Input: part model. Units: mm. Frame: model coordinates. Give positions to 0.01 mm unless a question says otherwise; leave off trailing zeros. Loops run counter-clockwise (first coordinate to the right, second up) from the corner with the lowest first, then second, coordinate; pieces in that order, holes last. Notation, with made-up numbers: M 16,18 L 47,18 A23 cw 47,57 Z; hole C 51,-10 d7. An arc over 180 degrees is marked long. One line per item, written item: value. Start each with the question number.
(1) Pin query (flat end, axial travel): P1, Ø11, axis at y = 314.18, z = 1303.08, coming from the -X side; P2, Ø4, axis at y = 259.2, z = 1328.48, coming from the -X side. Return the tip coordinate at first contact, or that it passes through.
(2) Section D-D on z = 1313.5. Output: boundary loops of the cut face in (x, y).
(3) Section C-C on y = 267.5. Output: boundary loops of the cut face in (x, z), plus the area to 3 significant figures.
(4) Section A-A on z = 1277. Output: boundary loops of the cut face in (x, y), plus the area to 3 significant figures.
(5) Section B-B on x = 95.3. Output: boundary loops of the cut face in (y, z) (3 decimals), plus the area to 3 significant figures.
(6) Ray query, line 1 along Z through (x, y) = (95.3, 316.5); line 2 along Y through (x, z) = (95.05, 1278.5); line 3 along Y through (x, z) = (94.45, 1280.5). Return the intervals inside material, ascending. Write a range as from..to.
(7) Pull-direction query (Z, two-part tool) for faces 1 (the cylindrical face through (94.479, 316.098, 1335.797)), 2 (the cylindrical face through (94.43, 284.75, 1325.1)), 3 (the flat face through (96.044, 298, 1310)); classes: released by +Z, released by -Z, zero draft, split by the parting line, or undercut.
```python
from build123d import *

# Parameters (mm, degrees)
BOSS_EXTRUDE1_START     = 92.868812
BOSS_EXTRUDE1_DEPTH     = 3.175
FILLET1_R               = 9.525
F_1_4_CLEARANCE_HOLE1_D = 6.7564


with BuildPart() as part:
    # Sketch1 → Boss-Extrude1 (new body)
    with BuildSketch(Plane(origin=(0, 0, 0), x_dir=(0, 0, -1), z_dir=(1, 0, 0)).offset(BOSS_EXTRUDE1_START)):
        with BuildLine():
            Line((-1304.620022056, 323.577914146), (-1279.556254241, 327.697081886))
            ThreePointArc((-1279.556254241, 327.697081886), (-1269.714759772, 322.976697122), (-1270.768280058, 312.11266745))
            Line((-1270.768280058, 312.11266745), (-1321.232047874, 253.01907305))
            ThreePointArc((-1321.232047874, 253.01907305), (-1331.771796135, 250.268190307), (-1338.000334154, 259.204574554))
            Line((-1338.000334154, 259.204574554), (-1338.000334154, 284.604574554))
            Line((-1338.000334154, 284.604574554), (-1338.000334154, 318.091943092))
            Line((-1338.000334154, 318.091943092), (-1304.620022056, 323.577914146))
        make_face()
    extrude(amount=BOSS_EXTRUDE1_DEPTH)

    # Fillet1
    fillet1_edges = [part.edges().sort_by_distance(p)[0] for p in [
        (94.456312, 318.091943092, 1338.000334154),
    ]]
    fillet(fillet1_edges, radius=FILLET1_R)

    # 1/4 Clearance Hole1 (through all)
    with Locations(Plane(origin=(96.043812484, 0, 0), x_dir=(0, 0, -1), z_dir=(1, 0, 0))):
        with Locations((-1303.075334154, 314.179001215), (-1278.011566338, 318.298168955), (-1328.475334154, 284.604574554), (-1328.475334154, 259.204574554)):
            Hole(F_1_4_CLEARANCE_HOLE1_D / 2)


solid = part.part
```
Output values:
1. P1: stops at x = 92.87
1. P2: passes through
2. outline: M 92.87,262.07 L 96.04,262.07 L 96.04,322.12 L 92.87,322.12 Z
3. outline: M 92.87,1308.87 L 96.04,1308.87 L 96.04,1338 L 92.87,1338 Z
3. area: 92.5 mm²
4. outline: M 92.87,304.82 L 96.04,304.82 L 96.04,315.07 L 92.87,315.07 Z; M 92.87,321.52 L 96.04,321.52 L 96.04,327.77 L 92.87,327.77 Z
4. area: 52.4 mm²
5. outline: M 253.019,1321.232 L 312.113,1270.768 A9.525 ccw 327.697,1279.556 L 319.403,1330.02 A9.525 ccw 310.005,1338 L 259.205,1338 A9.525 ccw Z; hole C 259.205,1328.475 d6.756; hole C 284.605,1328.475 d6.756; hole C 314.179,1303.075 d6.756; hole C 318.298,1278.012 d6.756
5. area: 3,130 mm²
6. line 1: z = 1268.66..1275.15, 1280.87..1300.62, 1305.53..1335.44
6. line 2: y = 303.06..314.96, 321.64..327.81
6. line 3: y = 300.72..316.01, 320.58..327.54
7. face 1: released by +Z
7. face 2: undercut
7. face 3: zero draft
